Can you work these out from the model? Positions are in its coordinate system, mm. A direction names the side the tool comes from. Give positions to 0.01 mm unless a question says otherwise; leave off trailing zeros. Loops run counter-clockwise (first coordinate to the right, second up) from the corner with the lowest first, then second, coordinate; pieces in that order, holes last. Notation, with made-up numbers: (-2, -35) -> (33, -35) arc R10 ccw to (33, -25) -> close; hole circle Ø10 at (82.25, 30.5). An arc over 180 degrees is marked (long way). One line per question, with ' | ' between items.
from build123d import *

# Parameters (mm, degrees)
F0_W     = 59.175328
F0_H     = 12.7
F1_DEPTH = 3.81


with BuildPart() as f1:
    # F0 (on Front) → F1 (new body)
    with BuildSketch(Plane.XZ):
        Polygon((81.28, 0), (0, 0), (0, -114.3), (0, -127), (0, -139.7), (81.28, -139.7), (81.28, -127), (81.28, -114.3), align=None)
        with Locations((40.643336, -120.65)):
            Rectangle(F0_W, F0_H, mode=Mode.SUBTRACT)
    extrude(amount=-F1_DEPTH)


solid = f1.part
Q1. On a 3-axis mill with a long thin cutter (end or side, diameter ignored), from which of +Z, -Z, +X, -X, +Y, -Y can I reach the whole of each face in a straight line? I mean faces 1 (the face through (81.28, 2, -71)), 2 (the face through (40, 2, -127)). Say none if no direction works.
Entries:
face 1: +Z, -Z, +X, +Y, -Y | face 2: +Y, -Y
Q2. If I drill on probe 1 along Z at (x, y) = (49, 1.5); probe 2 along X at (y, z) = (2.7, -118), over which ranges is the centre line in solid material (lowest first)? Write a range as from..to.
Entries:
probe 1: -139.7..-127, -114.3..0 | probe 2: 0..11.06, 70.23..81.28
Q3. If we section it at A-A (x = 26.5): Write out the boundary of the cut face in (y, z).
Entries:
outline: (0, -139.7) -> (3.81, -139.7) -> (3.81, -127) -> (0, -127) -> close; (0, -114.3) -> (3.81, -114.3) -> (3.81, 0) -> (0, 0) -> close
Q4. If we section it at B-B (y = 2.55): Write out the boundary of the cut face in (x, z), plus the area to 3 significant figures.
Entries:
outline: (0, -139.7) -> (81.28, -139.7) -> (81.28, 0) -> (0, 0) -> close; hole (11.06, -127) -> (70.23, -127) -> (70.23, -114.3) -> (11.06, -114.3) -> close | area: 10,600 mm²
Q5. If we mould it in two halves opening along Z, with no side actions, what happens to faces 3 (the face through (11.056, 2, -121)), 4 (the face through (40, 3.81, -69)), 5 (the face through (40, 2, -139.7))? For each: pulls with the +Z half, pulls with the -Z half, needs draft (parallel to the pull), parting line crosses it, or undercut.
Entries:
face 3: undercut | face 4: needs draft | face 5: pulls with the -Z half
